Check sheet for the modelled part. Datum: model origin and axes. Units: mm. A direction names the side the tool comes from. Give positions to 0.01 mm unless a question says otherwise; leave off trailing zeros. Loops run counter-clockwise (first coordinate to the right, second up) from the corner with the lowest first, then second, coordinate; pieces in that order, holes last. Notation, with made-up numbers: (44.5, 65) - (55.5, 65) arc R17 ccw to (55.5, 91) - close; hole circle Ø10 at (74, 45.25). An arc over 180 degrees is marked (long way). Answer in a Markdown table with one row per item. Add a question column.
(1) Sectioned sample at C-C on x = -7. Enter the section's corners in (y, z), then the cut area to 3 significant figures.
(2) Thickness scan on L1, parallel to X at y = 29.25, z = 9.5; L2, parallel to Y at x = 7, z = 23; L3, parallel to Y at x = 9, z = 10.5. Record the ranges inside material, lowest first.
(3) Sectioned sample at A-A on y = 20.5. Enter the section's corners in (x, z).
(4) Draft check along X on faces 1 (the face through (-16.43, 13.15, -18.9)), 2 (the face through (6.241, 6.583, 25.416)), 3 (the face through (-4, 13, 19.5)). Enter one of: released by +X, released by -X, zero draft, split by the parting line, or undercut.
(5) Sectioned sample at B-B on z = 9.5. Enter the section's corners in (x, y).
(6) Go/stop test with flat-tipped pins: P1, Ø4, axis at x = -7, z = 9.5, coming from the +Y side; P2, Ø4, axis at y = 24.5, z = 21, coming from the +X side; P3, Ø2, axis at x = 7.5, y = 10.5, coming from the +Z side; P4, Ø6.5, axis at x = 0, y = 12.5, coming from the +Z side. Record where each tip stops, or that it passes through.
(7) Sectioned sample at D-D on z = -4. Enter the section's corners in (x, y), then the cut area to 3 significant figures.
(8) Set-up check for faces 4 (the face through (7, 10, 19.5)), 5 (the face through (-7, 26, 9)), 6 (the face through (16.4, 13.15, 18.93)): record each of +Z, -Z, +X, -X, +Y, -Y from which the full face is reachable in a straight line by a thin tool's end or side.
from build123d import *

# Parameters (mm, degrees)
SKETCH1_W           = 34
SKETCH1_H           = 39
BOSS_EXTRUDE1_DEPTH = 26
SKETCH2_R           = 4.25
SKETCH2_R_2         = 3.5
BOSS_EXTRUDE2_DEPTH = 13
SKETCH3_R           = 4.25
SKETCH3_R_2         = 3.5
BOSS_EXTRUDE4_DEPTH = 12
FILLET1_R           = 2
FILLET3_R           = 2
SKETCH5_R           = 2.5
BOSS_EXTRUDE5_DEPTH = 2


with BuildPart() as part:
    # Sketch1 → Boss-Extrude1 (new body)
    with BuildSketch(Plane(origin=(0, 0, 0), x_dir=(1, 0, 0), z_dir=(0, 1, 0))):
        Rectangle(SKETCH1_W, SKETCH1_H)
    extrude(amount=BOSS_EXTRUDE1_DEPTH)

    # Sketch2 → Boss-Extrude2 (add)
    with BuildSketch(Plane(origin=(0, 26, 0), x_dir=(1, 0, 0), z_dir=(0, 1, 0))):
        with Locations(Location((-7, -9.5, 0), (0, 0, 90))):
            Circle(SKETCH2_R)
        with Locations(Location((-7, -9.5, 0), (0, 0, 90))):
            Circle(SKETCH2_R_2, mode=Mode.SUBTRACT)
    extrude(amount=BOSS_EXTRUDE2_DEPTH)

    # Sketch3 → Boss-Extrude4 (add)
    with BuildSketch(Plane.XY.offset(19.5)):
        with Locations(Location((7, 10, 0), (0, 0, 180))):
            Circle(SKETCH3_R)
        with Locations((7, 10)):
            Circle(SKETCH3_R_2, mode=Mode.SUBTRACT)
    extrude(amount=BOSS_EXTRUDE4_DEPTH)

    # Fillet1
    fillet1_edges = [part.edges().sort_by_distance(p)[0] for p in [
        (-17, 26, 0),
        (0, 26, 19.5),
        (17, 26, 0),
        (0, 0, 19.5),
        (-17, 0, 0),
        (0, 0, -19.5),
        (17, 0, 0),
        (17, 13, 19.5),
        (-17, 13, 19.5),
        (-17, 13, -19.5),
        (17, 13, -19.5),
        (0, 26, -19.5),
    ]]
    fillet(fillet1_edges, radius=FILLET1_R)

    # Fillet3
    fillet3_edges = [part.edges().sort_by_distance(p)[0] for p in [
        (-7, 26, 13.75),
        (11.25, 10, 19.5),
    ]]
    fillet(fillet3_edges, radius=FILLET3_R)

    # Sketch5 → Boss-Extrude5 (add)
    with BuildSketch(Plane.XZ):
        Polygon((-15, -6), (-15, 0), (-15, 6), (-27, 6), (-27, -6), align=None)
        with Locations((-22.5, 0)):
            Circle(SKETCH5_R, mode=Mode.SUBTRACT)
        Polygon((15, 6), (15, 0), (15, -6), (27, -6), (27, 6), align=None)
        with BuildLine():
            ThreePointArc((25, 0), (22.5, -2.5), (20, 0))
            ThreePointArc((20, 0), (22.5, 2.5), (25, 0))
        make_face(mode=Mode.SUBTRACT)
    extrude(amount=BOSS_EXTRUDE5_DEPTH)


with BuildPart() as boss_extrude5_kept_piece:
    # of the separate pieces the step leaves, the one the design keeps (boss_extrude5_pieces_kept)
    add(part.part.solids().sort_by_distance((0.75, 10, 19.5))[0])


solid = boss_extrude5_kept_piece.part
Reply:
| question | item | result |
|---|---|---|
| 1 | outline | (0, -17.5) arc R2 ccw to (2, -19.5) - (24, -19.5) arc R2 ccw to (26, -17.5) - (26, 3.25) arc R2 cw to (28, 5.25) - (39, 5.25) - (39, 6) - (26, 6) - (26, 13) - (39, 13) - (39, 13.75) - (28, 13.75) arc R2 cw to (26, 15.75) - (26, 17.5) arc R2 ccw to (24, 19.5) - (2, 19.5) arc R2 ccw to (0, 17.5) - close |
| 1 | area | 1,030 mm^2 |
| 2 | L1 | -11.25 to -10.5, -3.5 to -2.75 |
| 2 | L2 | 5.75 to 6.5, 13.5 to 14.25 |
| 2 | L3 | 0 to 26 |
| 3 | outline | (-17, -17.5) arc R2 ccw to (-15, -19.5) - (15, -19.5) arc R2 ccw to (17, -17.5) - (17, 17.5) arc R2 ccw to (15, 19.5) - (-15, 19.5) arc R2 ccw to (-17, 17.5) - close |
| 4 | face 1 | released by -X |
| 4 | face 2 | undercut |
| 4 | face 3 | zero draft |
| 5 | outline | (-17, 2) arc R2 ccw to (-15, 0) - (15, 0) arc R2 ccw to (17, 2) - (17, 24) arc R2 ccw to (15, 26) - (-0.75, 26) arc R2 cw to (-2.75, 28) - (-2.75, 39) - (-3.5, 39) - (-3.5, 26) - (-10.5, 26) - (-10.5, 39) - (-11.25, 39) - (-11.25, 28) arc R2 cw to (-13.25, 26) - (-15, 26) arc R2 ccw to (-17, 24) - close |
| 6 | P1 | y = 26 |
| 6 | P2 | x = 16.28 |
| 6 | P3 | z = 19.5 |
| 6 | P4 | z = 31.5 |
| 7 | outline | (-17, 2) arc R2 ccw to (-15, 0) - (15, 0) arc R2 ccw to (17, 2) - (17, 24) arc R2 ccw to (15, 26) - (-15, 26) arc R2 ccw to (-17, 24) - close |
| 7 | area | 881 mm^2 |
| 8 | face 4 | +Z |
| 8 | face 5 | +Y |
| 8 | face 6 | +Z, +X, +Y, -Y |
